Autodesk Fusion 360 part; units mm, degrees
sketch "スケッチ1" plane through (0, 0, 0) normal (0, 1, 0) x (1, 0, 0)
  circle A0 centre (0, 0) radius 210
  circle A1 centre (0, -210) radius 85
  line L0 (68.3017, -260.5952) -> (168.7454, -125)
  line L1 (-168.7454, -125) -> (-68.3017, -260.5952)
  circle A2 centre (0, -210) radius 77
  circle A3 centre (0, -210) radius 69
  line L2 (61.8733, -255.8333) -> (154.1352, -131.2832)
  line L3 (55.4449, -251.0714) -> (147.7068, -126.5213)
  line L4 (-61.8733, -255.8333) -> (-154.1352, -131.2832)
  line L5 (-147.7068, -126.5213) -> (-55.4449, -251.0714)
  circle A4 centre (154.1352, -131.2832) radius 8
  circle A5 centre (-154.1352, -131.2832) radius 8
  line L6 (0, -210) -> (0, -295)
  line L7 (-135, 0) -> (135, 0)
  line L8 (135, 0) -> (135, -155)
  line L9 (135, -155) -> (-135, -155)
  line L10 (-135, -155) -> (-135, 0)
  point P0 (0, -287)
  dimension "d1" = 420
  dimension "d2" = 170
  dimension "d3" = 210
  dimension "d4" = 155
  dimension "d5" = 16
  dimension "d13" = 270
  dimension "d14" = 155
extrude "押し出し1" add sketch "スケッチ1" along normal blind 5 contours A0 A5 | A0 A5 | A0 A1 L1 L4 A5 | A0 A4 | A0 A4 | A0 A1 L0 L2 A4 | A0 L4 A5 | A0 L4 L5 A5 L9 L10 | A1 A2 L4 L6 | A0 L2 A4 | A1 A2 L2 L6 | A0 A1 L4 L5 | A1 A2 L4 L5 | A0 A1 L2 L3 | A0 L2 L3 A4 L8 L9 | A1 A2 L2 L3 | A2 A3 L3 L6 | A2 A3 L5 L6
hole "穴1" at (0, 0, 287) at (-154.1352, 0, 131.2832) at (154.1352, 0, 131.2832) direction (0, 1, 0) diameter 3.2 end through all
fillet "フィレット1" radius 2 6 edges at (135, 2.5, 155) (-135, 2.5, 155) (126.6109, 2.5, 155) (135, 2.5, 143.675) (-135, 2.5, 143.675) (-126.6109, 2.5, 155)
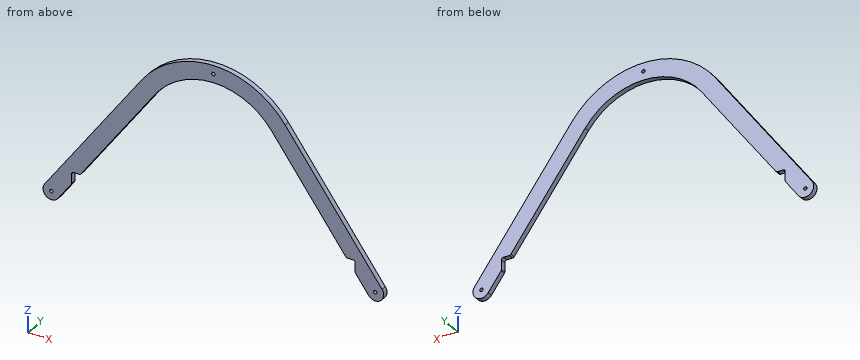
Read the model definition and answer for the solid it produces. Units are mm, in the model's axes. Coordinates: 2 decimals unless noted, no trailing zeros. Write each loop counter-clockwise with the first axis right and the second up, starting at its lowest first coordinate (ties: lowest second). Pieces come first, ordered by that corner, then holes. Notation, with made-up numbers: (13.5, -32.5) -> (23.5, -32.5) arc R7 ccw to (23.5, -23.5) -> close; hole circle Ø8 at (42.5, 81). An arc over 180 degrees is marked (long way). Write item = value, one per line.
(1) Straight lines are drawn through the part: L1, parallel to Z at x = 0, y = 3.8; L2, parallel to X at y = 4.55, z = 155.5; L3, parallel to X at y = 4.75, z = 228. For each, find the intervals that lie inside material, in ascending order. Write a range as from..to.
From the geometry:
L1 = 279..285.4, 288.6..295
L2 = -146.15..-126.3, 126.3..146.15
L3 = -92.45..-72.54, 72.54..92.45
(2) Section A-A on z = 272 is taken. Write down the section's boundary in (x, y), plus the area to 3 significant figures.
From the geometry:
outline = (-58.15, 0) -> (-30.28, 0) -> (-30.28, 5) -> (-58.15, 5) -> close; (30.28, 0) -> (58.15, 0) -> (58.15, 5) -> (30.28, 5) -> close
area = 279 mm2
(3) Given pin 1 Ø1.5 at (y, z) = (3, 148) entering from -X; pin 2 Ø2 at (x, y) = (12.5, 3) entering from +Z; pin 3 Ø2 at (y, z) = (3.5, 189) entering from -X, each flat-ended and moving along its own axis, determine where each tip first touches the part or whether it passes through.
From the geometry:
pin_1 = -152.26
pin_2 = 294.22
pin_3 = -122.08
(4) Section B-B on y = 3.7 is taken. Write down the section's boundary in (x, z).
From the geometry:
outline = (-160.56, 136.05) arc R8 ccw to (-147.71, 126.52) -> (-135.39, 143.14) arc R2 ccw to (-135, 144.34) -> (-135, 153) arc R2 cw to (-133, 155) -> (-127.62, 155) arc R2 ccw to (-126.01, 155.81) -> (-55.44, 251.07) arc R69 cw to (55.44, 251.07) -> (126.01, 155.81) arc R2 ccw to (127.62, 155) -> (133, 155) arc R2 cw to (135, 153) -> (135, 144.34) arc R2 ccw to (135.39, 143.14) -> (147.71, 126.52) arc R8 ccw to (160.56, 136.05) -> (68.3, 260.6) arc R85 ccw to (-68.3, 260.6) -> close; hole circle Ø3.2 at (-154.14, 131.28); hole circle Ø3.2 at (0, 287); hole circle Ø3.2 at (154.14, 131.28)
(5) Section C-C on z = 150 is taken. Write down the section's boundary in (x, y), plus the area to 3 significant figures.
From the geometry:
outline = (-150.23, 0) -> (-135, 0) -> (-135, 5) -> (-150.23, 5) -> close; (135, 0) -> (150.23, 0) -> (150.23, 5) -> (135, 5) -> close
area = 152 mm2
(6) Section D-D on x = 138.5 is taken. Write down the section's boundary in (y, z).
From the geometry:
outline = (0, 138.95) -> (5, 138.95) -> (5, 165.83) -> (0, 165.83) -> close
